from build123d import *

# Parameters (mm, degrees)
SKETCH2_R               = 3
BOSS_EXTRUDE1_DEPTH     = 25
CUT_EXTRUDE1_DEPTH      = 26.357444666
CUT_EXTRUDE1_DEPTH_BACK = 26.357444666
SKETCH3_R               = 0.75
FILLET1_R               = 0.5


with BuildPart() as part:
    # Sketch2 → Boss-Extrude1 (new body)
    with BuildSketch(Plane.XY):
        Circle(SKETCH2_R)
    extrude(amount=BOSS_EXTRUDE1_DEPTH)

    # Sketch3 → Cut-Extrude1 (cut, two sides: drawn at the far end of the back side and taken through both)
    with BuildSketch(Plane(origin=(0, 0, 0), x_dir=(1, 0, 0), z_dir=(0, 1, 0)).offset(-CUT_EXTRUDE1_DEPTH_BACK)):
        with Locations(Location((0, -5, 0), (0, 0, 270))):
            Circle(SKETCH3_R)
    extrude(amount=CUT_EXTRUDE1_DEPTH + CUT_EXTRUDE1_DEPTH_BACK, mode=Mode.SUBTRACT)

    # Fillet1
    fillet1_edges = [part.edges().sort_by_distance(p)[0] for p in [
        (-3, 0, 0),
    ]]
    fillet(fillet1_edges, radius=FILLET1_R)


solid = part.part
Verification items for the finished model (mm, model axes). Coordinates: 2 decimals unless noted, no trailing zeros. Loops run counter-clockwise (first coordinate to the right, second up) from the corner with the lowest first, then second, coordinate; pieces in that order, holes last. Notation, with made-up numbers: (62, 25) -> (66, 25) arc R13 cw to (66, 46) -> close; hole circle Ø3 at (22, 73). An arc over 180 degrees is marked (long way). Answer as CSV lines item,"result".
1) Thickness scan on L1, parallel to Z at x = 0, y = -0.25; L2, parallel to Z at x = -0.5, y = 1; L3, parallel to X at y = 1, z = 5. Record the ranges inside material, lowest first. Write a range as from..to.
Found:
L1,"z = 0..4.25, 5.75..25"
L2,"z = 0..4.44, 5.56..25"
L3,"x = -2.83..-0.75, 0.75..2.83"
2) Release check for a two-part mould opening along Z. For faces 1 (the flat face through (0, 0, 25)), 2 (the cylindrical face through (-0.65, -2.93, 12.58)), 3 (the cylindrical face through (0.03, -0.04, 4.25)) record: +Z half, -Z half, draft (parallel to the pull), parting line (faces both ways), or undercut.
Found:
face 1,"+Z half"
face 2,"draft"
face 3,"undercut"
3) Depth check by flat-ended pin: pin 1 (1.5 mm diameter, centred on y = -1.5, z = 12.5, fed in from +X); pin 2 (1.2 mm diameter, centred on x = 0, z = 5, fed in from -Y); pin 3 (1 mm diameter, centred on x = -1, z = 8, fed in from -Y); pin 4 (1 mm diameter, centred on x = 2, y = 0, fed in from -Z). Enter the tip coordinate at first touch or a pass-through.
Found:
pin 1,"stops at x = 2.9"
pin 2,"passes through"
pin 3,"stops at y = -2.96"
pin 4,"stops at z = 0"
4) Cross-section at B-B, the plane z = 12.5. Record the cut outline in (x, y), then the cut area to 3 significant figures.
Found:
outline,"circle Ø6 at (0, 0)"
area,"28.3 mm2"
5) Cross-section at A-A, the plane x = 0. Record the cut outline in (y, z), then the cut area to 3 significant figures.
Found:
outline,"(-3, 0.5) arc R0.5 ccw to (-2.5, 0) -> (2.5, 0) arc R0.5 ccw to (3, 0.5) -> (3, 4.25) -> (-3, 4.25) -> close; (-3, 5.75) -> (3, 5.75) -> (3, 25) -> (-3, 25) -> close"
area,"141 mm2"
6) Cross-section at C-C, the plane z = 5. Record the cut outline in (x, y).
Found:
outline,"(-0.75, -2.9) -> (-0.75, 2.9) arc R3 ccw to start; (0.75, -2.9) arc R3 ccw to (0.75, 2.9) -> close"
